The model under review builds one solid part; all positions refer to its coordinate system, in mm. Face numbers are marked on the shaded views. Give positions to 0.01 mm unless a question says otherwise; leave off trailing zeros. Loops run counter-clockwise (first coordinate to the right, second up) from the corner with the lowest first, then second, coordinate; pieces in that order, holes last. Notation, with made-up numbers: (-38.75, -26.5) - (-28.75, -26.5) arc R15 cw to (-28.75, 2.5) - close; hole circle Ø10 at (-27.75, 14). An arc over 180 degrees is marked (long way). Answer as a JSON object with one key per item and string values.
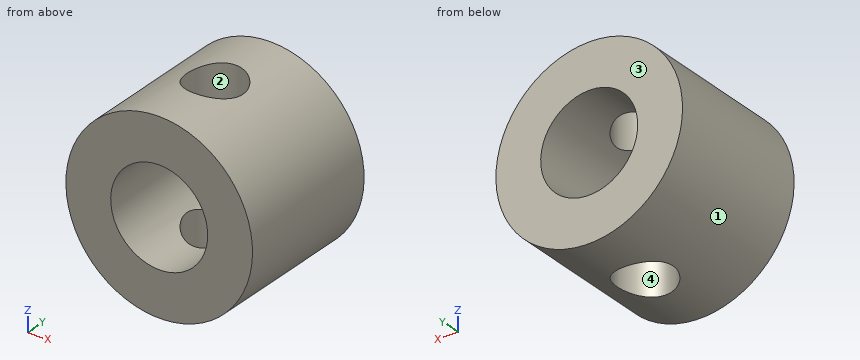
from build123d import *

# Parameters (mm, degrees)
SKETCH1_R           = 5
BOSS_EXTRUDE1_DEPTH = 8
SKETCH2_R           = 2.6
CUT_EXTRUDE1_DEPTH  = 20
SKETCH3_R           = 1.5
CUT_EXTRUDE2_DEPTH  = 20


with BuildPart() as part:
    # Sketch1 → Boss-Extrude1 (new body)
    with BuildSketch(Plane(origin=(0, 0, 0), x_dir=(1, 0, 0), z_dir=(0, 1, 0))):
        with Locations(Location((0, 0, 0), (0, 0, 270))):
            Circle(SKETCH1_R)
    extrude(amount=BOSS_EXTRUDE1_DEPTH)

    # Sketch2 → Cut-Extrude1 (cut, symmetric)
    with BuildSketch(Plane(origin=(0, 0, 0), x_dir=(1, 0, 0), z_dir=(0, 1, 0))):
        with Locations(Location((0, 0, 0), (0, 0, 270))):
            Circle(SKETCH2_R)
    extrude(amount=CUT_EXTRUDE1_DEPTH, both=True, mode=Mode.SUBTRACT)

    # Sketch3 → Cut-Extrude2 (cut, symmetric)
    with BuildSketch(Plane.XY):
        with Locations((0, 4)):
            Circle(SKETCH3_R)
    extrude(amount=CUT_EXTRUDE2_DEPTH, both=True, mode=Mode.SUBTRACT)


solid = part.part
Q1. Clearance check with flat-ended pins moving along their axes: pin 1 Ø1 at (y, z) = (5.5, 4) entering from +X; pin 2 Ø2 at (x, y) = (1.5, 4) entering from -Z; pin 3 Ø4 at (x, z) = (0, 0) entering from -Y. State where each tip first meets the part, or that it passes through.
Results:
{"pin 1": "stops at x = 3.57", "pin 2": "stops at z = -4.86", "pin 3": "passes through"}
Q2. To check wall thickness, follow probe 1 along Y at (x, z) = (0, 4); probe 2 along X at (y, z) = (2, 0); probe 3 along X at (y, z) = (2.75, 1). State the ranges of each line that lie inside material, in increasing order. Write a range as [from, to].
Results:
{"probe 1": "y = [0, 2.5], [5.5, 8]", "probe 2": "x = [-5, -2.6], [2.6, 5]", "probe 3": "x = [-4.9, -2.4], [2.4, 4.9]"}
Q3. Consider section A-A, the plane x = 0. State the section outline as (y, z) points, plus the area to 3 significant figures.
Results:
{"outline": "(0, -5) - (2.5, -5) - (2.5, -2.6) - (0, -2.6) - close; (0, 2.6) - (2.5, 2.6) - (2.5, 5) - (0, 5) - close; (5.5, -5) - (8, -5) - (8, -2.6) - (5.5, -2.6) - close; (5.5, 2.6) - (8, 2.6) - (8, 5) - (5.5, 5) - close", "area": "24.0 mm^2"}
Q4. Consider section D-D, the plane x = -4. State the section outline as (y, z) points, plus the area to 3 significant figures.
Results:
{"outline": "(0, -3) - (8, -3) - (8, 3) - (0, 3) - close", "area": "48.0 mm^2"}
Q5. The part is to be moulded in two halves that separate along X. For the marked faces 1, 2, 3 and 4, say which applies: +X half, -X half, draft (parallel to the pull), parting line (faces both ways), or undercut.
Results:
{"face 1": "parting line", "face 2": "undercut", "face 3": "draft", "face 4": "undercut"}
Q6. Consider section C-C, the plane y = 5. State the section outline as (x, z) points.
Results:
{"outline": "(-1.12, -4.87) - (-1.12, -2.35) arc R2.6 cw to (-1.12, 2.35) - (-1.12, 4.87) arc R5 ccw to start; (1.12, -4.87) arc R5 ccw to (1.12, 4.87) - (1.12, 2.35) arc R2.6 cw to (1.12, -2.35) - close"}
Q7. Consider section B-B, the plane z = 0. State the section outline as (x, y) points, plus the area to 3 significant figures.
Results:
{"outline": "(-5, 0) - (-2.6, 0) - (-2.6, 8) - (-5, 8) - close; (2.6, 0) - (5, 0) - (5, 8) - (2.6, 8) - close", "area": "38.4 mm^2"}
